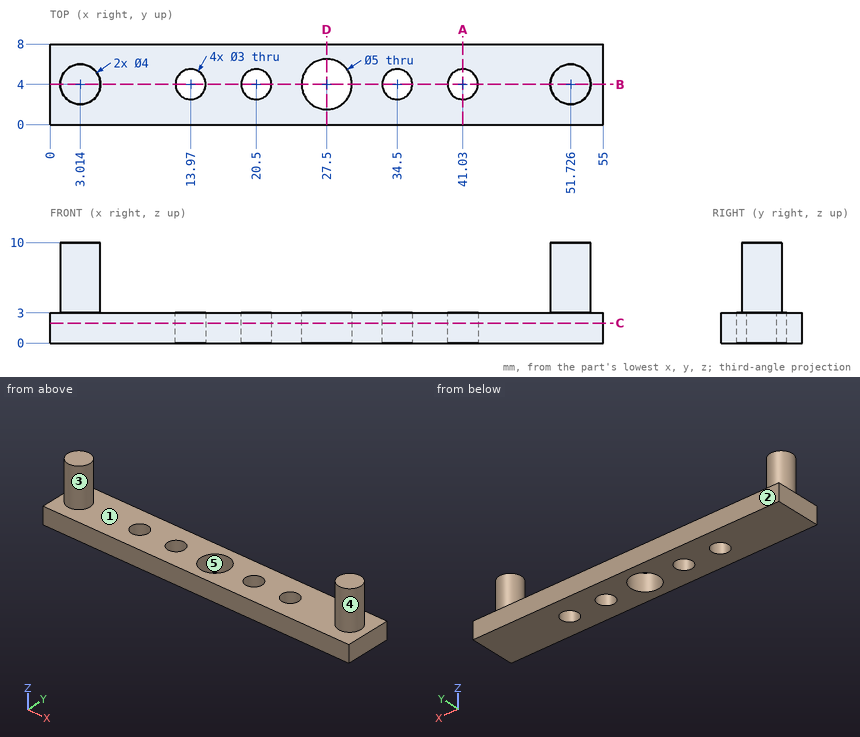
Input: dimensioned drawing with shaded views. Units: mm. Origin: part minimum x, y, z. A direction names the side the tool comes from. Round coordinates to 2 decimals unless told otherwise and drop trailing zeros. Order: outer loops, then holes, each group sorted by start corner. A loop starts at its lowest first (then second) coordinate and runs counter-clockwise, first axis right, second up.
1. Mould query, pull axis X, two halves, no side actions, for the marked faces 1, 2 and 3. Classes: released by +X, released by -X, zero draft, split by the parting line, or undercut.
The answers:
face 1: undercut
face 2: zero draft
face 3: undercut
2. Cut plane C-C, the plane z = 2. Output: boundary loops of the cut face in (x, y), then the cut area to 3 significant figures.
The answers:
outline: (0, 0) - (55, 0) - (55, 8) - (0, 8) - close; hole circle Ø3 at (13.97, 4); hole circle Ø3 at (20.5, 4); hole circle Ø5 at (27.5, 4); hole circle Ø3 at (34.5, 4); hole circle Ø3 at (41.03, 4)
area: 392 mm2
3. Cut plane A-A, the plane x = 41.03. Output: boundary loops of the cut face in (y, z), then the cut area to 3 significant figures.
The answers:
outline: (0, 0) - (2.5, 0) - (2.5, 3) - (0, 3) - close; (5.5, 0) - (8, 0) - (8, 3) - (5.5, 3) - close
area: 15.0 mm2
4. Pin query (flat end, axial travel): P1, Ø2, axis at y = 3, z = 7.5, coming from the +X side; P2, Ø1.5, axis at x = 18.5, y = 4.5, coming from the -Z side. Return the tip coordinate at first contact, or that it passes through.
The answers:
P1: stops at x = 53.73
P2: stops at z = 0
5. Set-up query: the marked faces 4 and 5. Return all of +Z, -Z, +X, -X, +Y, -Y with unobstructed straight access to the full face (end or side cutting, diameter ignored); none if empty.
The answers:
face 4: +Z
face 5: +Z, -Z
6. Cut plane B-B, the plane y = 4. State how many separate pieces and enclosed holes the cut face has, then the cut area to 3 significant figures.
The answers:
separate pieces: 6
enclosed holes: 0
area: 170 mm2
7. Material intervals for line 1 (Y direction, x = 20.5, z = 0.7); line 2 (Y direction, x = 27.5, z = 1.85); line 3 (Z direction, x = 8.5, y = 5), sorted ascending.
The answers:
line 1: y = 0 to 2.5, 5.5 to 8
line 2: y = 0 to 1.5, 6.5 to 8
line 3: z = 0 to 3
8. Cut plane D-D, the plane x = 27.5. Output: boundary loops of the cut face in (y, z), then the cut area to 3 significant figures.
The answers:
outline: (0, 0) - (1.5, 0) - (1.5, 3) - (0, 3) - close; (6.5, 0) - (8, 0) - (8, 3) - (6.5, 3) - close
area: 9.00 mm2
